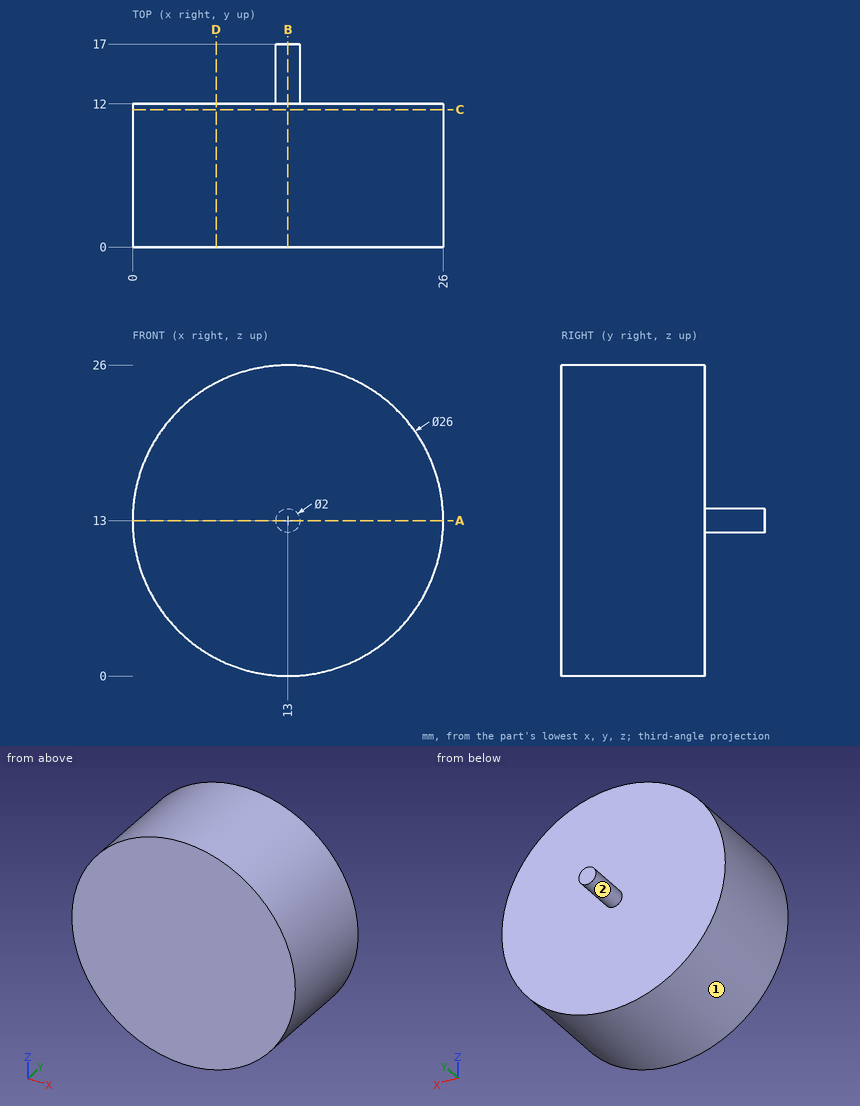
Part print with two shaded views. Sizes in mm from the minimum x, y, z corner. A direction names the side the tool comes from. Round coordinates to 2 decimals unless told otherwise and drop trailing zeros. Order: outer loops, then holes, each group sorted by start corner. A loop starts at its lowest first (then second) coordinate and runs counter-clockwise, first axis right, second up.
(1) Band-saw the part on C-C (y = 11.5). List the corners of the cut face in (x, z).
(2) Band-saw the part on D-D (x = 7). List the corners of the cut face in (y, z).
(3) Pin check, flat tips, straight feed: pin 1 (5 mm diameter, centred on y = 11.5, z = 6, fed in from +X); pin 2 (12 mm diameter, centred on x = 7.5, z = 20.5, fed in from +Y); pin 3 (3 mm diameter, centred on y = 10, z = 20, fed in from -X). Stop position of each tip, or through.
(4) Band-saw the part on A-A (z = 13). List the corners of the cut face in (x, y).
(5) Band-saw the part on B-B (x = 13). List the corners of the cut face in (y, z), then the cut area to 3 significant figures.
(6) 3-axis set-ups, long thin cutter, end or side, ignore diameter. For the marked faces 1 and 2: which of +Z, -Z, +X, -X, +Y, -Y reach the whole face in a straight line?
(7) Drill centre lines: line 1 (Y direction, x = 6.25, z = 11.5); line 2 (Z direction, x = 19.75, y = 11.75); line 3 (Z direction, x = 25, y = 10). Where is each one in solid material? Low to high.
Verdict:
1. outline: circle Ø26 at (13, 13)
2. outline: (0, 1.47) - (12, 1.47) - (12, 24.53) - (0, 24.53) - close
3. pin 1: stops at x = 25.2
3. pin 2: stops at y = 12
3. pin 3: stops at x = 1.22
4. outline: (0, 0) - (26, 0) - (26, 12) - (14, 12) - (14, 17) - (12, 17) - (12, 12) - (0, 12) - close
5. outline: (0, 0) - (12, 0) - (12, 12) - (17, 12) - (17, 14) - (12, 14) - (12, 26) - (0, 26) - close
5. area: 322 mm2
6. face 1: +Y, -Y
6. face 2: +Y
7. line 1: y = 0 to 12
7. line 2: z = 1.89 to 24.11
7. line 3: z = 8 to 18
